from build123d import *

# Parameters (mm, degrees)
SKETCH1_R           = 49.276
SKETCH1_R_2         = 6.5024
SKETCH1_R_3         = 12.7
BOSS_EXTRUDE1_DEPTH = 9.525
SKETCH2_R           = 49.276
SKETCH2_R_2         = 44.45
BOSS_EXTRUDE2_DEPTH = 63.5
SKETCH3_R           = 12.7
SKETCH3_R_2         = 6.5024
BOSS_EXTRUDE3_DEPTH = 15.875
CHAMFER1_SIZE       = 6.35
CHAMFER1_SIZE2      = 2.54
SKETCH4_R           = 12.7
BOSS_EXTRUDE4_DEPTH = 6.35
FILLET1_R           = 2.54


with BuildPart() as part:
    # Sketch1 → Boss-Extrude1 (new body)
    with BuildSketch(Plane(origin=(0, 0, 0), x_dir=(1, 0, 0), z_dir=(0, 1, 0))):
        Circle(SKETCH1_R)
        Circle(SKETCH1_R_2, mode=Mode.SUBTRACT)
        with Locations((0, 28.575)):
            Circle(SKETCH1_R_3, mode=Mode.SUBTRACT)
        with Locations((27.176439953, 8.830160614)):
            Circle(SKETCH1_R_3, mode=Mode.SUBTRACT)
        with Locations((16.795963584, -23.117660614)):
            Circle(SKETCH1_R_3, mode=Mode.SUBTRACT)
        with Locations((-16.795963584, -23.117660614)):
            Circle(SKETCH1_R_3, mode=Mode.SUBTRACT)
        with Locations((-27.176439953, 8.830160614)):
            Circle(SKETCH1_R_3, mode=Mode.SUBTRACT)
    extrude(amount=BOSS_EXTRUDE1_DEPTH)

    # Sketch2 → Boss-Extrude2 (add)
    with BuildSketch(Plane(origin=(0, 9.525, 0), x_dir=(1, 0, 0), z_dir=(0, 1, 0))):
        Circle(SKETCH2_R)
        Circle(SKETCH2_R_2, mode=Mode.SUBTRACT)
    extrude(amount=BOSS_EXTRUDE2_DEPTH)

    # Sketch3 → Boss-Extrude3 (add)
    with BuildSketch(Plane(origin=(0, 9.525, 0), x_dir=(1, 0, 0), z_dir=(0, 1, 0))):
        Circle(SKETCH3_R)
        Circle(SKETCH3_R_2, mode=Mode.SUBTRACT)
    extrude(amount=BOSS_EXTRUDE3_DEPTH)

    # Chamfer1
    chamfer1_edges = [part.edges().sort_by_distance(p)[0] for p in [
        (-49.276, 73.025, 0),
    ]]
    chamfer1_side = [part.faces().sort_by_distance(p)[0] for p in [
        (-49.276, 36.5125, 0),
    ]]
    chamfer(chamfer1_edges, length=CHAMFER1_SIZE, length2=CHAMFER1_SIZE2, reference=chamfer1_side[0])

    # Sketch4 → Boss-Extrude4 (add)
    with BuildSketch(Plane(origin=(0, 25.4, 0), x_dir=(1, 0, 0), z_dir=(0, 1, 0))):
        Circle(SKETCH4_R)
    extrude(amount=BOSS_EXTRUDE4_DEPTH)

    # Fillet1
    fillet1_edges = [part.edges().sort_by_distance(p)[0] for p in [
        (-12.7, 31.75, 0),
    ]]
    fillet(fillet1_edges, radius=FILLET1_R)


solid = part.part
Geometry check sheet. Reference: the model listing, model coordinates, mm. A direction names the side the tool comes from. Give positions to 0.01 mm unless a question says otherwise; leave off trailing zeros. Write each loop counter-clockwise with the first axis right and the second up, starting at its lowest first coordinate (ties: lowest second). Pieces come first, ordered by that corner, then holes.
1) Release check for a two-part mould opening along Z. For faces 1 (the face through (21.62, 72.72, 41.57)), 2 (the face through (-0.846, 12.522, -6.447)), 3 (the face through (10, 0, -1)) record: released by +Z, released by -Z, zero draft, split by the parting line, or undercut.
Values follow:
face 1: split by the parting line
face 2: undercut
face 3: zero draft
2) Go/stop test with flat-tipped pins: pin 1 Ø1 at (y, z) = (36.5, -28.5) entering from +X; pin 2 Ø1.5 at (x, y) = (-8.5, 25.5) entering from +Z; pin 3 Ø4 at (y, z) = (62, -5) entering from +X. Record where each tip stops, or that it passes through.
Values follow:
pin 1: stops at x = 40.55
pin 2: stops at z = 48.66
pin 3: stops at x = 49.18
3) Cross-section at A-A (z = 0). Record the boundary of the cut face in (x, y) (3 decimals).
Values follow:
outline: (-49.276, 0) - (-36.304, 0) - (-36.304, 9.525) - (-44.45, 9.525) - (-44.45, 73.025) - (-46.736, 73.025) - (-49.276, 66.675) - close; (-18.049, 0) - (-6.502, 0) - (-6.502, 25.4) - (6.502, 25.4) - (6.502, 0) - (18.049, 0) - (18.049, 9.525) - (12.7, 9.525) - (12.7, 29.21) arc R2.54 ccw to (10.16, 31.75) - (-10.16, 31.75) arc R2.54 ccw to (-12.7, 29.21) - (-12.7, 9.525) - (-18.049, 9.525) - close; (36.304, 0) - (49.276, 0) - (49.276, 66.675) - (46.736, 73.025) - (44.45, 73.025) - (44.45, 9.525) - (36.304, 9.525) - close
4) Cross-section at C-C (z = -18). Count the separate pieces of the cut face and the enclosed holes in it, plus the area to 3 significant figures.
Values follow:
separate pieces: 4
enclosed holes: 0
area: 1,050 mm2
5) Cross-section at B-B (x = 0). Record the boundary of the cut face in (y, z) (3 decimals), plus the area to 3 significant figures.
Values follow:
outline: (0, -49.276) - (66.675, -49.276) - (73.025, -46.736) - (73.025, -44.45) - (9.525, -44.45) - (9.525, -41.275) - (0, -41.275) - close; (0, -15.875) - (9.525, -15.875) - (9.525, -12.7) - (29.21, -12.7) arc R2.54 ccw to (31.75, -10.16) - (31.75, 10.16) arc R2.54 ccw to (29.21, 12.7) - (9.525, 12.7) - (9.525, 44.45) - (73.025, 44.45) - (73.025, 46.736) - (66.675, 49.276) - (0, 49.276) - (0, 6.502) - (25.4, 6.502) - (25.4, -6.502) - (0, -6.502) - close
area: 1,520 mm2
6) Set-up check for faces 4 (the face through (0, 25.4, 0)), 5 (the face through (17.1, 4.7, -1.1)), 6 (the face through (9.3, 9.525, 9.3)): record each of +Z, -Z, +X, -X, +Y, -Y from which the full face is reachable in a straight line by a thin tool's end or side.
Values follow:
face 4: -Y
face 5: +Y, -Y
face 6: +Y
7) Thickness scan on line 1 (Z direction, x = 0, y = 3) (3 decimals); line 2 (X direction, y = 15, z = -0.5); line 3 (Z direction, x = 2, y = 4). Record the ranges inside material, lowest first.
Values follow:
line 1: z = -49.276 to -41.275, -15.875 to -6.502, 6.502 to 49.276
line 2: x = -49.27 to -44.45, -12.69 to -6.48, 6.48 to 12.69, 44.45 to 49.27
line 3: z = -49.24 to -41.12, -16.03 to -6.19, 6.19 to 49.24
